Autodesk Fusion 360 part; units mm, degrees
sketch "Sketch1" plane through (0, 0, 0) normal (1, 0, 0) x (0, 1, 0)
  circle A0 centre (0, 0) radius 0.5
  line L0 (0.325, -0.325) -> (-0.325, -0.325)
  line L1 (-0.325, -0.325) -> (-0.325, 0.325)
  line L2 (-0.325, 0.325) -> (0.325, 0.325)
  line L3 (0.325, 0.325) -> (0.325, -0.325)
  line L4 (0.325, -0.325) -> (-0.325, 0.325) construction
  line L5 (-0.325, -0.325) -> (0.325, 0.325) construction
  dimension "d1" = 1
  dimension "d2" = 0.65
  dimension "d3" = 0.65
extrude "Extrude1" add sketch "Sketch1" along normal blind 54 contours A0 | L0 L1 L2 L3
sketch "Sketch2" plane through (54, 0, 0) normal (1, 0, 0) x (0, 1, 0)
  circle A0 centre (0, 0) radius 0.5
  line L0 (0.325, -0.325) -> (-0.325, -0.325)
  line L1 (-0.325, -0.325) -> (-0.325, 0.325)
  line L2 (-0.325, 0.325) -> (0.325, 0.325)
  line L3 (0.325, 0.325) -> (0.325, -0.325)
  line L4 (0.325, -0.325) -> (-0.325, 0.325) construction
  line L5 (-0.325, -0.325) -> (0.325, 0.325) construction
  dimension "d8" = 0.65
  dimension "d9" = 0.65
extrude "Extrude2" add sketch "Sketch2" along normal blind 1.265 contours L0 L1 L2 L3
extrude "Extrude3" add sketch "Sketch1" against normal blind 1.265 contours L0 L1 L2 L3
sketch "Sketch3" plane through (0, 0, -0.325) normal (0, 0, -1) x (1, 0, 0)
  line L0 (54, 0.325) -> (54, -0.325)
  line L1 (54, -0.325) -> (55.265, -0.325)
  line L2 (55.265, -0.325) -> (55.265, 0.325)
  line L3 (55.265, 0.325) -> (54, 0.325)
  line L4 (55.265, 0.325) -> (54.615, 0.325)
  line L5 (54.615, 0.325) -> (54.615, -0.325)
  line L6 (54.615, -0.325) -> (55.265, -0.325)
  line L7 (55.265, -0.325) -> (55.265, 0.325)
  line L8 (55.265, 0.325) -> (54.615, -0.325) construction
  line L9 (54.615, 0.325) -> (55.265, -0.325) construction
  point P0 (54.94, 0)
  dimension "d14" = 0.65
  dimension "d15" = 0.65
sketch "Sketch4" plane through (0, 0, -0.325) normal (0, 0, -1) x (1, 0, 0)
  line L0 (0, -0.325) -> (0, 0.325)
  line L1 (0, 0.325) -> (-1.265, 0.325)
  line L2 (-1.265, 0.325) -> (-1.265, -0.325)
  line L3 (-1.265, -0.325) -> (0, -0.325)
  line L4 (-0.615, -0.325) -> (-1.265, -0.325)
  line L5 (-1.265, -0.325) -> (-1.265, 0.325)
  line L6 (-1.265, 0.325) -> (-0.615, 0.325)
  line L7 (-0.615, 0.325) -> (-0.615, -0.325)
  line L8 (-0.615, -0.325) -> (-1.265, 0.325) construction
  line L9 (-1.265, -0.325) -> (-0.615, 0.325) construction
  point P0 (-0.94, 0)
  dimension "d17" = 0.65
  dimension "d18" = 0.65
extrude "Extrude4" add sketch "Sketch4" sketch "Sketch3" along normal blind 2.75 contours L1 L2 L3 L4 L5 L6 L7 of sketch 2 contours L1 L2 L3 L4 L5 L6 L7
fillet "Fillet1" radius 0.5 2 edges at (-0.615, 0, -0.325) (54.615, 0, -0.325)
fillet "Fillet2" radius 1 2 edges at (-1.265, 0, 0.325) (55.265, 0, 0.325)
fillet "Fillet3" radius 0.2 28 edges at (-0.94, -0.325, -3.075) (-0.615, 0, -3.075) (-0.94, 0.325, -3.075) (-1.265, 0, -3.075) (-0.4686, -0.325, -0.4714) (-0.615, -0.325, -1.95) (-0.1325, -0.325, 0.325) (-0.9721, -0.325, 0.0321) (-1.265, -0.325, -1.875) (-0.1325, 0.325, 0.325) (-0.9721, 0.325, 0.0321) (-1.265, 0.325, -1.875) (-0.4686, 0.325, -0.4714) (-0.615, 0.325, -1.95) (54.1325, -0.325, 0.325) (54.9721, -0.325, 0.0321) (55.265, -0.325, -1.875) (54.615, -0.325, -1.95) (54.4686, -0.325, -0.4714) (55.265, 0.325, -1.875) (54.9721, 0.325, 0.0321) (54.1325, 0.325, 0.325) (54.4686, 0.325, -0.4714) (54.615, 0.325, -1.95) (54.94, 0.325, -3.075) (55.265, 0, -3.075) (54.94, -0.325, -3.075) (54.615, 0, -3.075)
equation "d1 = width"
equation "d2 = d3"
equation "d3 = d1 * 0.65"
equation "width = 1 mm"
equation "baseLenght = 54 mm"
equation "d6 = baseLenght"
equation "d8 = width * 0.65"
equation "d9 = d8"
equation "d14 = width * 0.65"
equation "d15 = d14"
equation "d17 = width * 0.65"
equation "d18 = d17"
equation "d26 = 0.2 * width"
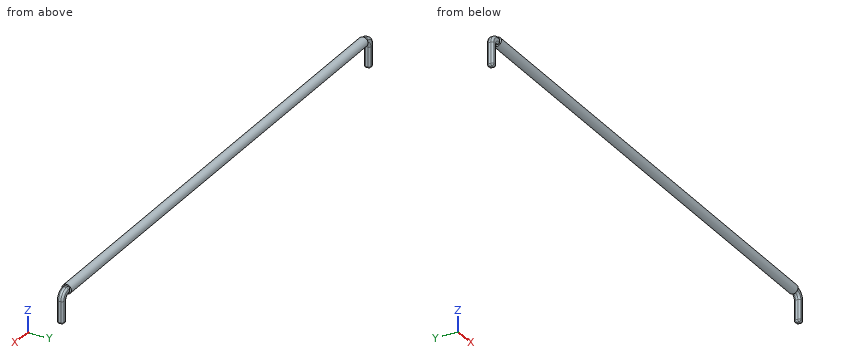
Source: CAD feature listing. Evaluate the final solid. Frame: model axes, mm. Coordinates: 2 decimals unless noted, no trailing zeros. Loops run counter-clockwise (first coordinate to the right, second up) from the corner with the lowest first, then second, coordinate; pieces in that order, holes last. Notation, with made-up numbers: (-26.5, 22) -> (-3.5, 22) arc R18 cw to (-3.5, 54) -> close; hole circle Ø5 at (44, 84). An arc over 180 degrees is marked (long way). Answer in a Markdown table with one row per item. Add a question column.
Q1. Section B-B on x = 23.5. Return the cut outline in (y, z), and give its area (3 significant figures).
Q2. Contact query for flat-ended pins moving along their axis: pin 1 Ø0.5 at (y, z) = (0, 0) entering from -X; pin 2 Ø0.9 at (x, z) = (-0.5, -2) entering from +Y (3 decimals); pin 3 Ø0.5 at (y, z) = (0, 0) entering from +X. Output: stop coordinate, or through.
Q3. Ray query, line 1 along X through (y, z) = (0.15, -2.2); line 2 along X through (y, z) = (-0.25, -0.15); line 3 along Z through (x, y) = (51, 0.05). Return the intervals inside material, ascending.
Q4. Section A-A on z = -1.6. Return the cut outline in (x, y) (3 decimals), and give its area (3 significant figures).
Computed values:
| question | item | result |
|---|---|---|
| 1 | outline | circle Ø1 at (0, 0) |
| 1 | area | 0.785 mm^2 |
| 2 | pin 1 | stops at x = -1.17 |
| 2 | pin 2 | stops at y = 0.325 |
| 2 | pin 3 | stops at x = 55.17 |
| 3 | line 1 | x = -1.26 to -0.62, 54.62 to 55.26 |
| 3 | line 2 | x = -1.06 to 55.06 |
| 3 | line 3 | z = -0.5 to 0.5 |
| 4 | outline | (-1.265, -0.125) arc R0.2 ccw to (-1.065, -0.325) -> (-0.815, -0.325) arc R0.2 ccw to (-0.615, -0.125) -> (-0.615, 0.125) arc R0.2 ccw to (-0.815, 0.325) -> (-1.065, 0.325) arc R0.2 ccw to (-1.265, 0.125) -> close; (54.615, -0.125) arc R0.2 ccw to (54.815, -0.325) -> (55.065, -0.325) arc R0.2 ccw to (55.265, -0.125) -> (55.265, 0.125) arc R0.2 ccw to (55.065, 0.325) -> (54.815, 0.325) arc R0.2 ccw to (54.615, 0.125) -> close |
| 4 | area | 0.776 mm^2 |
